Drawing for the job (mm, zero at the part's lowest x, y, z). A direction names the side the tool comes from. Give positions to 0.01 mm unless a question says otherwise; leave off trailing zeros. Loops run counter-clockwise (first coordinate to the right, second up) from the corner with the lowest first, then second, coordinate; pieces in that order, holes last.
1) 3-axis set-ups, long thin cutter, end or side, ignore diameter. For the marked faces 1 and 2: which of +Z, -Z, +X, -X, +Y, -Y reach the whole face in a straight line?
2) Band-saw the part on C-C on y = 15.2. List the corners of the cut face in (x, z), then the cut area to 3 significant figures.
3) Band-saw the part on A-A on x = 16. List the corners of the cut face in (y, z), then the cut area to 3 significant figures.
4) Band-saw the part on B-B on z = 31. List the corners of the cut face in (x, y).
5) Band-saw the part on D-D on z = 4.5. List the corners of the cut face in (x, y).
6) Flat gauge pins, fed straight in: P1, Ø2, axis at x = 17, z = 17.5, coming from the -Y side; P2, Ø1, axis at x = 6.5, y = 7.5, coming from the +Z side; P3, Ø3.5, axis at x = 4, z = 31, coming from the -Y side. Where does each tip first touch, or does it go through?
7) Wall check: line 1 (Y direction, x = 10, z = 4.5); line 2 (Z direction, x = 16, y = 22.7); line 3 (Y direction, x = 9.25, z = 2). Give the ranges that are in metal, low to high.
8) Two-plate mould, pull along X, no slides. Class the marked faces 3, 4 and 5: +X half, -X half, draft (parallel to the pull), parting line (faces both ways), or undercut.
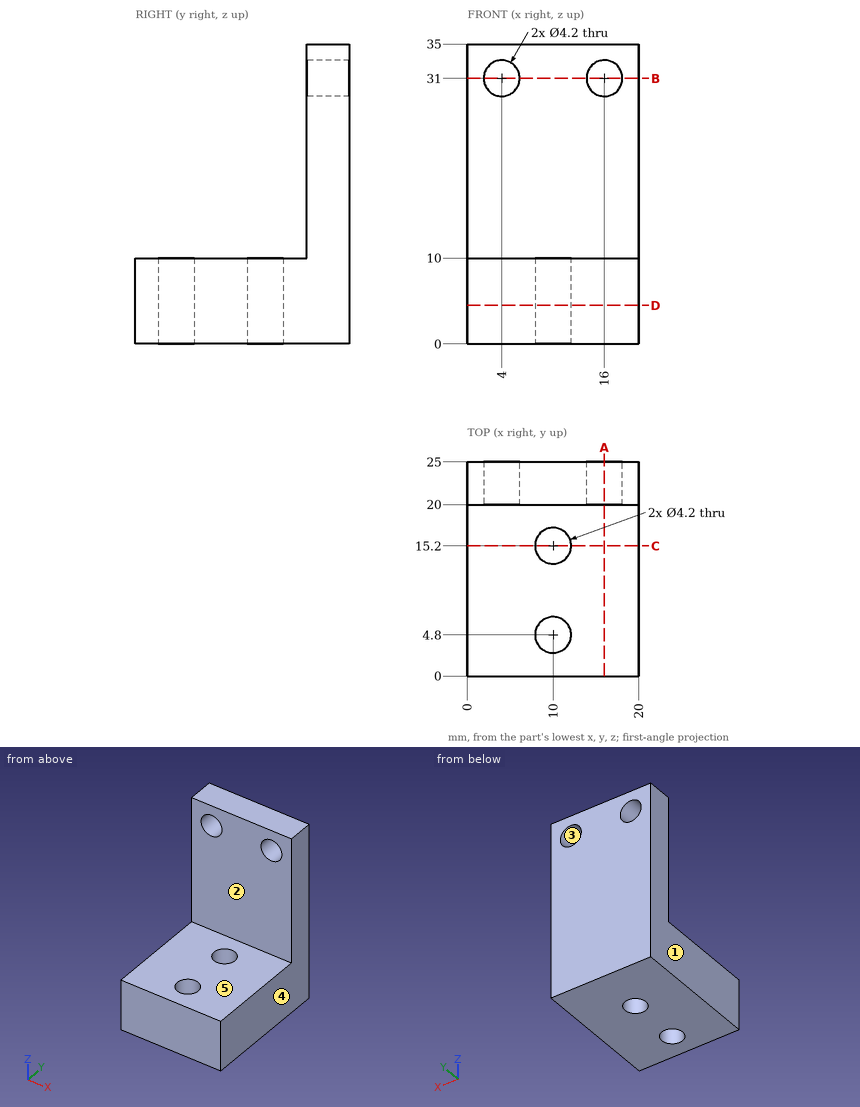
Findings below:
1. face 1: +Z, -Z, -X, +Y, -Y
1. face 2: +Z, +X, -X, -Y
2. outline: (0, 0) - (7.9, 0) - (7.9, 10) - (0, 10) - close; (12.1, 0) - (20, 0) - (20, 10) - (12.1, 10) - close
2. area: 158 mm2
3. outline: (0, 0) - (25, 0) - (25, 28.9) - (20, 28.9) - (20, 10) - (0, 10) - close; (20, 33.1) - (25, 33.1) - (25, 35) - (20, 35) - close
3. area: 354 mm2
4. outline: (0, 20) - (1.9, 20) - (1.9, 25) - (0, 25) - close; (6.1, 20) - (13.9, 20) - (13.9, 25) - (6.1, 25) - close; (18.1, 20) - (20, 20) - (20, 25) - (18.1, 25) - close
5. outline: (0, 0) - (20, 0) - (20, 25) - (0, 25) - close; hole circle Ø4.2 at (10, 4.8); hole circle Ø4.2 at (10, 15.2)
6. P1: stops at y = 20
6. P2: stops at z = 10
6. P3: passes through
7. line 1: y = 0 to 2.7, 6.9 to 13.1, 17.3 to 25
7. line 2: z = 0 to 28.9, 33.1 to 35
7. line 3: y = 0 to 2.84, 6.76 to 13.24, 17.16 to 25
8. face 3: undercut
8. face 4: +X half
8. face 5: draft
